Can you work these out from the model? Positions are in its coordinate system, mm. Give positions to 0.01 mm unless a question says otherwise; leave off trailing zeros. Write each loop counter-clockwise with the first axis right and the second up, starting at its lowest first coordinate (ties: lowest second). Pieces come first, ordered by that corner, then holes. Notation, with made-up numbers: M 51.5,-14 L 94.5,-14 A34 cw 94.5,17 Z; hole C 70.5,-16 d2. An arc over 180 degrees is marked long. Write each question's results on one line, items separated by ' | '.
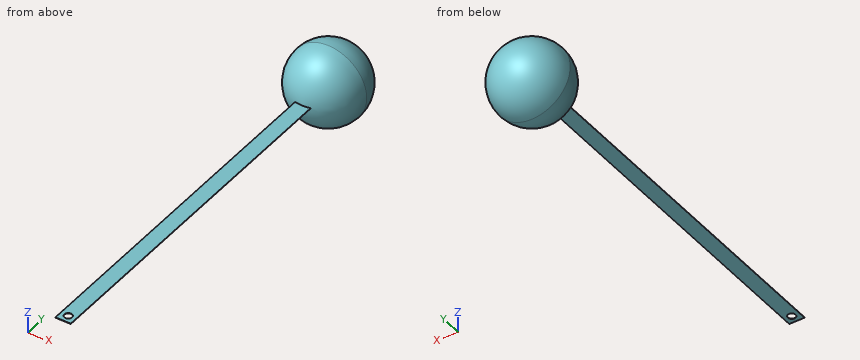
from build123d import *

# Parameters (mm, degrees)
BOSS_EXTRUDE2_REACH      = 566.447
BOSS_EXTRUDE2_END_RADIUS = 50
SKETCH6_W                = 20
SKETCH6_H                = 0.5
CUT_EXTRUDE1_DEPTH       = 565.468832178
CUT_EXTRUDE1_DEPTH_BACK  = 565.468832178
SKETCH7_R                = 5


with BuildPart() as part:
    # Sketch1 one side → Revolve3 (revolve)
    with BuildSketch(Plane.XY):
        with BuildLine():
            ThreePointArc((0, 460), (35.355339059, 474.644660941), (50, 510))
            ThreePointArc((50, 510), (35.355339059, 545.355339059), (0, 560))
            Line((0, 560), (0, 460))
        make_face()
    revolve(axis=Axis((0, 510, 0), (0, -1, 0)))

    # Boss-Extrude2: up to this sphere (the profile starts outside it)
    boss_extrude2_end = Location((0, 510, 0)) * Sphere(BOSS_EXTRUDE2_END_RADIUS, mode=Mode.PRIVATE)
    # Sketch6 → Boss-Extrude2 (add, up to the surface)
    with BuildSketch(Plane(origin=(0, 0, 0), x_dir=(1, 0, 0), z_dir=(0, 1, 0)), mode=Mode.PRIVATE) as boss_extrude2_sk1:
        Rectangle(SKETCH6_W, SKETCH6_H)
    boss_extrude2_tool1 = extrude(boss_extrude2_sk1.sketch, amount=BOSS_EXTRUDE2_REACH, mode=Mode.PRIVATE) - boss_extrude2_end
    add(boss_extrude2_tool1.solids().sort_by_distance((0, 0, 0))[0])

    # Sketch7 → Cut-Extrude1 (cut, two sides: drawn at the far end of the back side and taken through both)
    with BuildSketch(Plane.XY.offset(0.25).offset(-CUT_EXTRUDE1_DEPTH_BACK)):
        with Locations((0, 10)):
            Circle(SKETCH7_R)
    extrude(amount=CUT_EXTRUDE1_DEPTH + CUT_EXTRUDE1_DEPTH_BACK, mode=Mode.SUBTRACT)


solid = part.part
Item 1: I'm going to push flat-ended pins straight in: pin 1 (22 mm diameter, centred on x = 3.5, y = 277, fed in from -Z); pin 2 (1 mm diameter, centred on x = -16, z = -4.5, fed in from +Y); pin 3 (2 mm diameter, centred on x = 4, z = 39, fed in from +Y); pin 4 (8 mm diameter, centred on x = 0, y = 10, fed in from +Z). Where does each tip first touch, or does it pass through?
Geometry says:
pin 1: stops at z = -0.25 | pin 2: stops at y = 557.33 | pin 3: stops at y = 542.26 | pin 4: passes through
Item 2: I want a section at B-B, the plane x = 0. Please give me the cut outline in (y, z).
Geometry says:
outline: M 0,-0.25 L 5,-0.25 L 5,0.25 L 0,0.25 Z; M 15,-0.25 L 460,-0.25 A50 ccw long 460,0.25 L 15,0.25 Z
Item 3: I want a section at C-C, the plane y = 244.5. Please give me the cut outline in (x, z).
Geometry says:
outline: M -10,-0.25 L 10,-0.25 L 10,0.25 L -10,0.25 Z
Item 4: If I drill on line 1 (X direction, y = 10, z = 0.15); line 2 (Z direction, x = 5.5, y = 236.5); line 3 (X direction, y = 158.5, z = 0), over which ranges is the centre line in solid material (lowest first)? Write a range as from..to.
Geometry says:
line 1: x = -10..-5, 5..10 | line 2: z = -0.25..0.25 | line 3: x = -10..10
Item 5: I want a section at A-A, the plane y = 10. Please give me the cut outline in (x, z).
Geometry says:
outline: M -10,-0.25 L -5,-0.25 L -5,0.25 L -10,0.25 Z; M 5,-0.25 L 10,-0.25 L 10,0.25 L 5,0.25 Z
Item 6: I want a section at D-D, the plane z = 27. Please give me the cut outline in (x, y), and give its area (3 significant figures).
Geometry says:
outline: C 0,510 d84.17 | area: 5,560 mm2
